Read the model definition and answer for the solid it produces. Units are mm, in the model's axes. Face numbers are marked on the shaded views. A direction names the side the tool comes from. Coordinates: 2 decimals unless noted, no trailing zeros. Loops run counter-clockwise (first coordinate to the right, second up) from the corner with the lowest first, then second, coordinate; pieces in that order, holes last. Notation, with made-up numbers: (-3, 30) - (34, 30) arc R15 cw to (34, 43) - close; hole circle Ø7 at (18, -36.5). An arc over 180 degrees is marked (long way). Use CSV: the item, a comma, the result in double quotes.
Autodesk Inventor part; units mm, degrees
ref_plane "YZ Plane" through (0, 0, 0) normal (1, 0, 0) x (0, 1, 0)
ref_plane "XZ Plane" through (0, 0, 0) normal (0, 1, 0) x (-1, 0, 0)
ref_plane "XY Plane" through (0, 0, 0) normal (0, 0, 1) x (1, 0, 0)
sketch "Sketch1" plane through (0, 0, 0) normal (0, 0, 1) x (1, 0, 0)
  line L0 (37.5, 0) -> (37.5, 30)
  line L1 (37.5, 30) -> (22.1407, 42)
  line L2 (22.1407, 42) -> (-22.1407, 42)
  line L3 (-22.1407, 42) -> (-37.5, 30)
  line L4 (-37.5, 30) -> (-37.5, 0)
  circle A0 centre (-28.678, 21) radius 3.5
  circle A1 centre (28.678, 21) radius 3.5
  circle A2 centre (0, 21) radius 3.75
  line L5 (-37.5, 0) -> (-25, 0)
  line L6 (-25, 0) -> (-25, 3.2)
  line L7 (-25, 3.2) -> (25, 3.2)
  line L8 (25, 3.2) -> (25, 0)
  line L9 (25, 0) -> (37.5, 0)
  line L10 (0, -8.4) -> (0, 50.4)
  line L11 (-52.5, 0) -> (52.5, 0)
  point P0 (0, 0)
  point P1 (0, 42)
  point P2 (0, 0)
  dimension "d0" = 30
  dimension "d1" = 30
  dimension "d3" = 128
  dimension "d4" = 75
  dimension "d5" = 7
  dimension "d7" = 7
  dimension "d9" = 28.678
  dimension "d10" = 28.678
  dimension "d24" = 7.5
  dimension "d28" = 50
  dimension "d29" = 12.5
  dimension "d30" = 3.2
  dimension "d31" = 37.5
  dimension "d32" = 128
  dimension "d33" = 3.2
  dimension "d34" = 17.8
  dimension "d36" = 44.2814
extrude "Extrusion2" add sketch "Sketch1" along normal blind 6 contours L9 L8 L7 L10 A2 L2 L1 L0 | L10 A2 L7 L6 L5 L4 L3 L2
fillet "Fillet2" radius 6 4 edges at (-22.1407, 42, 3) (22.1407, 42, 3) (37.5, 30, 3) (-37.5, 30, 3)
equation "\"d1\" = d0"
equation "\"d7\" = d5"
properties part number "Tope riel final"
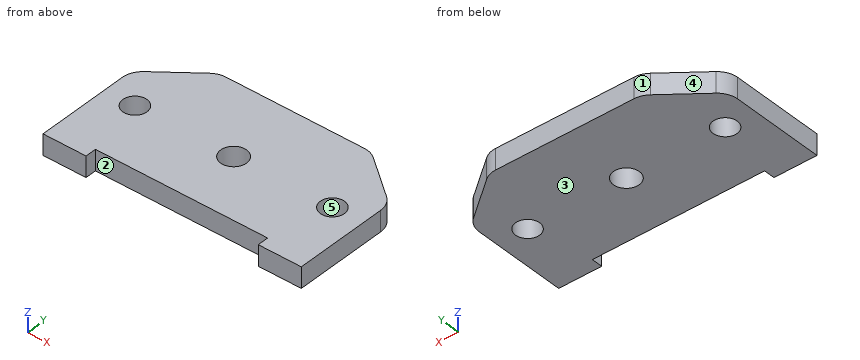
Q1. Find the intervals of material crossed by probe 1 along Y at (x, z) = (7.5, 5.55); probe 2 along X at (y, z) = (19, 4.75); probe 3 along Y at (x, z) = (-30.5, 4.6), in increasing order. Write a range as [from, to].
Reported:
probe 1,"y = [3.2, 42]"
probe 2,"x = [-37.5, -31.55], [-25.81, -3.17], [3.17, 25.81], [31.55, 37.5]"
probe 3,"y = [0, 18.01], [23.99, 35.47]"
Q2. A tool of negligible diameter and unlimited length cuts with its end or side. For the marked faces 1 and 2, from which of +Z, -Z, +X, -X, +Y, -Y can it reach the whole face along a straight path? Write none if from no direction.
Reported:
face 1,"+Z, -Z, -X, +Y"
face 2,"+Z, -Z, -Y"
Q3. For a pull along X with two mould halves and no side action, classify the marked faces 3, 4 and 5 as +X half, -X half, draft (parallel to the pull), parting line (faces both ways), or undercut.
Reported:
face 3,"draft"
face 4,"-X half"
face 5,"undercut"
Q4. The part is cut by section C-C on z = 5.25. Determine the outline of the cut face in (x, y), and give its area (3 significant figures).
Reported:
outline,"(-37.5, 0) - (-25, 0) - (-25, 3.2) - (25, 3.2) - (25, 0) - (37.5, 0) - (37.5, 27.07) arc R6 ccw to (35.19, 31.8) - (23.77, 40.73) arc R6 ccw to (20.07, 42) - (-20.07, 42) arc R6 ccw to (-23.77, 40.73) - (-35.19, 31.8) arc R6 ccw to (-37.5, 27.07) - close; hole circle Ø7 at (-28.68, 21); hole circle Ø7.5 at (0, 21); hole circle Ø7 at (28.68, 21)"
area,"2,680 mm²"
Q5. The part is cut by section D-D on y = 37. Determine the outline of the cut face in (x, z).
Reported:
outline,"(-28.54, 0) - (28.54, 0) - (28.54, 6) - (-28.54, 6) - close"
Q6. The part is cut by section B-B on y = 21. Determine the outline of the cut face in (x, z), and give its area (3 significant figures).
Reported:
outline,"(-37.5, 0) - (-32.18, 0) - (-32.18, 6) - (-37.5, 6) - close; (-25.18, 0) - (-3.75, 0) - (-3.75, 6) - (-25.18, 6) - close; (3.75, 0) - (25.18, 0) - (25.18, 6) - (3.75, 6) - close; (32.18, 0) - (37.5, 0) - (37.5, 6) - (32.18, 6) - close"
area,"321 mm²"
Q7. The part is cut by section A-A on x = 0. Determine the outline of the cut face in (y, z).
Reported:
outline,"(3.2, 0) - (17.25, 0) - (17.25, 6) - (3.2, 6) - close; (24.75, 0) - (42, 0) - (42, 6) - (24.75, 6) - close"
